Input: part model. Units: mm. Frame: model coordinates. A direction names the side the tool comes from. Coordinates: 2 decimals unless noted, no trailing zeros. Write each loop counter-clockwise with the first axis right and the second up, starting at its lowest first coordinate (ties: lowest second). Pieces come first, ordered by that corner, then holes. Notation, with made-up numbers: (81.5, -10) -> (93.5, -10) arc R22 cw to (93.5, 7) -> close; hole circle Ø6 at (25.25, 70). An arc over 180 degrees is marked (long way). One line per question, with ' | ' between items. Start each with the question number.
```python
from build123d import *

# Parameters (mm, degrees)
SKETCH_1_R          = 1.9
SKETCH_1_R_2        = 2
EXTRUDE_1_DEPTH     = 35
EXTRUDE_2_DEPTH     = 35
CUT_EXTRUDE_1_DEPTH = 118.156356153
SKETCH_4_R          = 41.5
CUT_EXTRUDE_2_DEPTH = 5.5
SKETCH_5_R          = 31
CUT_EXTRUDE_3_DEPTH = 116.632442624


with BuildPart() as part:
    # 草图1 → 凸台-拉伸1 (new body)
    with BuildSketch(Plane.XY):
        with BuildLine():
            Line((-46.419972715, 26.434696638), (-100.702636481, 42))
            Line((-100.702636481, 42), (-100.702636481, 48))
            Line((-100.702636481, 48), (100.702636481, 48))
            Line((100.702636481, 48), (100.702636481, 42))
            Line((100.702636481, 42), (46.419972715, 26.434696638))
            ThreePointArc((46.419972715, 26.434696638), (35.478614393, 20.327525063), (28.382623085, 10))
            Line((28.382623085, 10), (-28.382623085, 10))
            ThreePointArc((-28.382623085, 10), (-35.478614393, 20.327525063), (-46.419972715, 26.434696638))
        make_face()
        with Locations((-54, 37)):
            Circle(SKETCH_1_R, mode=Mode.SUBTRACT)
        with Locations((-35.5, 32.04293994)):
            Circle(SKETCH_1_R, mode=Mode.SUBTRACT)
        with Locations((-21.95706006, 18.5)):
            Circle(SKETCH_1_R, mode=Mode.SUBTRACT)
        with Locations(Location((21.95706006, 18.5, 0), (0, 0, 180))):
            Circle(SKETCH_1_R, mode=Mode.SUBTRACT)
        with Locations(Location((35.5, 32.04293994, 0), (0, 0, 180))):
            Circle(SKETCH_1_R, mode=Mode.SUBTRACT)
        with Locations(Location((54, 37, 0), (0, 0, 180))):
            Circle(SKETCH_1_R, mode=Mode.SUBTRACT)
        with Locations((-90, 44)):
            Circle(SKETCH_1_R_2, mode=Mode.SUBTRACT)
        with Locations((-70, 44)):
            Circle(SKETCH_1_R_2, mode=Mode.SUBTRACT)
        with Locations(Location((70, 44, 0), (0, 0, 180))):
            Circle(SKETCH_1_R_2, mode=Mode.SUBTRACT)
        with Locations(Location((90, 44, 0), (0, 0, 180))):
            Circle(SKETCH_1_R_2, mode=Mode.SUBTRACT)
    extrude(amount=EXTRUDE_1_DEPTH)

    # 草图2 → 凸台-拉伸2 (add)
    with BuildSketch(Plane.XY.offset(35)):
        Polygon((-100.702636481, 42), (-100.978273837, 41.038738304), (-67.334114479, 31.39143085), (-67.058477124, 32.352692546), align=None)
        Polygon((67.058477124, 32.352692546), (100.702636481, 42), (100.978273837, 41.038738304), (67.334114479, 31.39143085), align=None)
    extrude(amount=-EXTRUDE_2_DEPTH)

    # 草图3 → 切除-拉伸1 (cut, through all)
    with BuildSketch(Plane.XY.offset(35)):
        with BuildLine():
            Line((-6.641746516, 40.210125207), (-15.476556882, 19.658485028))
            ThreePointArc((-15.476556882, 19.658485028), (-17.211519663, 18.450985714), (-19.06092662, 19.474628401))
            ThreePointArc((-19.06092662, 19.474628401), (-30.09691848, 32.072460053), (-45.323396591, 39.047619048))
            ThreePointArc((-45.323396591, 39.047619048), (-46.877626016, 41.21821789), (-44.889566421, 43))
            Line((-44.889566421, 43), (-8.479162585, 43))
            ThreePointArc((-8.479162585, 43), (-6.808870756, 42.100056911), (-6.641746516, 40.210125207))
        make_face()
        with BuildLine():
            Line((-10.837416069, 17.789874793), (-1.837416069, 38.725781047))
            ThreePointArc((-1.837416069, 38.725781047), (0, 39.935906254), (1.837416069, 38.725781047))
            Line((1.837416069, 38.725781047), (10.837416069, 17.789874793))
            ThreePointArc((10.837416069, 17.789874793), (10.670291829, 15.899943089), (9, 15))
            Line((9, 15), (-9, 15))
            ThreePointArc((-9, 15), (-10.670291829, 15.899943089), (-10.837416069, 17.789874793))
        make_face()
        with BuildLine():
            Line((44.889566421, 43), (8.479162585, 43))
            ThreePointArc((8.479162585, 43), (6.808870756, 42.100056911), (6.641746516, 40.210125207))
            Line((6.641746516, 40.210125207), (15.476556882, 19.658485028))
            ThreePointArc((15.476556882, 19.658485028), (17.211519663, 18.450985714), (19.06092662, 19.474628401))
            ThreePointArc((19.06092662, 19.474628401), (30.09691848, 32.072460053), (45.323396591, 39.047619048))
            ThreePointArc((45.323396591, 39.047619048), (46.877626016, 41.21821789), (44.889566421, 43))
        make_face()
    extrude(amount=-CUT_EXTRUDE_1_DEPTH, mode=Mode.SUBTRACT)

    # 草图4 → 切除-拉伸2 (cut)
    with BuildSketch(Plane(origin=(0, 0, 0), x_dir=(-1, 0, 0), z_dir=(0, 0, -1))):
        with Locations((54, 0)):
            Circle(SKETCH_4_R)
        with Locations((-54, 0)):
            Circle(SKETCH_4_R)
    extrude(amount=-CUT_EXTRUDE_2_DEPTH, mode=Mode.SUBTRACT)

    # 草图5 → 切除-拉伸3 (cut, through all)
    with BuildSketch(Plane(origin=(0, 0, 5.5), x_dir=(-1, 0, 0), z_dir=(0, 0, -1))):
        with Locations((-54, 0)):
            Circle(SKETCH_5_R)
        with Locations((54, 0)):
            Circle(SKETCH_5_R)
    extrude(amount=-CUT_EXTRUDE_3_DEPTH, mode=Mode.SUBTRACT)


solid = part.part
```
1) Section B-B, the plane y = 37. Return loops of the section in (x, z).
2) Section C-C, the plane y = 13. Return loops of the section in (x, z), then the cut area to 3 significant figures.
3) Pull-direction query (X, two-part tool) for faces 6 (the face through (69.077, 45.774, 17.255)), 7 (the face through (15.033, 14.277, 2.712)), 8 (the face through (-1, 48, 17)); classes: released by +X, released by -X, zero draft, split by the parting line, or undercut.
4) Section D-D, the plane x = 58. Return loops of the section in (y, z).
5) First-contact query: P1, Ø1.8, axis at y = 44.5, z = 20.5, coming from the +X side; P2, Ø2, axis at x = 40, z = 15, coming from the -Y side; P3, Ø9.5, axis at x = -48, y = 28, coming from the -Z side. Flat tips, straight axial feed; report the tip coordinate or a pass-through.
6) Access query for faces 1 (the face through (62.6, 40.6, 2.7)), 2 (the face through (27, 43, 18)), 3 (the face through (38.3, 26.73, 20.04)), 4 (the face through (100.703, 45, 17)), 5 (the face through (-1, 42, 35)). Directions: +Z, -Z, +X, -X, +Y, -Y. A direction counts if a zero-diameter tool reaches every point of the face in a straight line with its end or side. Return the directions, or none.
7) Ray query, line 1 (Y direction, x = 22.5, z = 9); line 2 (Y direction, x = 54, z = 23); line 3 (Y direction, x = 23, z = 6). Return the intervals inside material, ascending.
8) Section A-A, the plane x = -54. Return loops of the section in (y, z), then the cut area to 3 significant figures.
Answer block:
1) outline: (-86.89, 0) -> (-72.79, 0) -> (-72.79, 5.5) -> (-55.9, 5.5) -> (-55.9, 35) -> (-86.89, 35) -> close; (-52.1, 5.5) -> (-38.8, 5.5) -> (-38.8, 35) -> (-52.1, 35) -> close; (-8.02, 0) -> (-2.58, 0) -> (-2.58, 35) -> (-8.02, 35) -> close; (2.58, 0) -> (8.02, 0) -> (8.02, 35) -> (2.58, 35) -> close; (38.8, 5.5) -> (52.1, 5.5) -> (52.1, 35) -> (38.8, 35) -> close; (55.9, 5.5) -> (72.79, 5.5) -> (72.79, 0) -> (86.89, 0) -> (86.89, 35) -> (55.9, 35) -> close
2) outline: (-25.86, 5.5) -> (-14.59, 5.5) -> (-14.59, 0) -> (14.59, 0) -> (14.59, 5.5) -> (25.86, 5.5) -> (25.86, 35) -> (-25.86, 35) -> close | area: 1,690 mm2
3) face 6: undercut | face 7: released by +X | face 8: zero draft
4) outline: (30.74, 5.5) -> (41.31, 5.5) -> (41.31, 0) -> (48, 0) -> (48, 35) -> (30.74, 35) -> close
5) P1: stops at x = 100.7 | P2: stops at y = 27.13 | P3: stops at z = 5.5
6) face 1: -Z, -Y | face 2: +Z, -Z | face 3: +Z, -Z, -Y | face 4: +Z, -Z, +X, +Y | face 5: +Z, +X, -X, +Y, -Y
7) line 1: y = 10 to 16.68, 20.32 to 24.65, 43 to 48 | line 2: y = 31 to 35.1, 38.9 to 48 | line 3: y = 10 to 16.91, 20.09 to 25.28, 43 to 48
8) outline: (31, 5.5) -> (35.1, 5.5) -> (35.1, 35) -> (31, 35) -> close; (38.9, 5.5) -> (41.5, 5.5) -> (41.5, 0) -> (48, 0) -> (48, 35) -> (38.9, 35) -> close | area: 425 mm2
